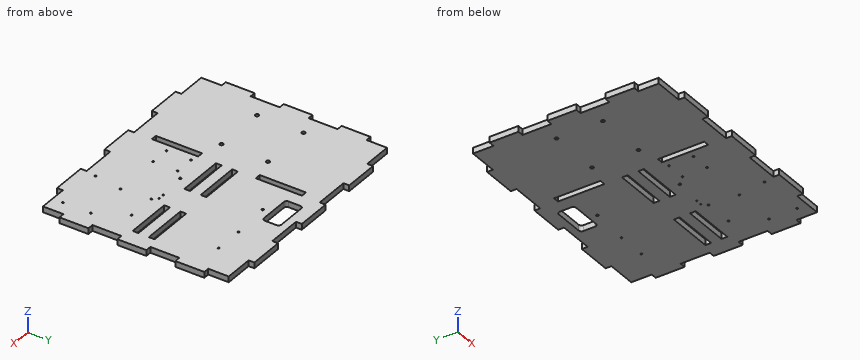
```python
from build123d import *

# Parameters (mm, degrees)
SKETCH_W        = 10
SKETCH_H        = 79.8
SKETCH_W_2      = 79.8
SKETCH_H_2      = 10
PAD_DEPTH       = 10
SKETCH001_R     = 3
POCKET_DEPTH    = 10.001
SKETCH002_R     = 1.5
POCKET001_DEPTH = 10.001
SKETCH003_R     = 1.5
POCKET002_DEPTH = 10.001
SKETCH004_R     = 2
POCKET003_DEPTH = 10.001
POCKET004_DEPTH = 10.001
SKETCH006_R     = 1.2
POCKET005_DEPTH = 10.001
SKETCH007_R     = 1.5
POCKET006_DEPTH = 10.001


with BuildPart() as part:
    # Sketch → Pad (new body)
    with BuildSketch(Plane.XY):
        Polygon((0, 0), (0, 35.3), (-10, 35.3), (-10, 85.1), (0, 85.1), (0, 135.1), (-10, 135.1), (-10, 184.9), (0, 184.9), (0, 234.9), (-10, 234.9), (-10, 284.7), (0, 284.7), (0, 320), (50.2, 320), (50.2, 330), (110.2, 330), (110.2, 320), (170.2, 320), (170.2, 330), (230.2, 330), (230.2, 320), (290.2, 320), (290.2, 330), (350.2, 330), (350.2, 320), (400.4, 320), (400.4, 284.7), (410.4, 284.7), (410.4, 234.9), (400.4, 234.9), (400.4, 184.9), (410.4, 184.9), (410.4, 135.1), (400.4, 135.1), (400.4, 85.1), (410.4, 85.1), (410.4, 35.3), (400.4, 35.3), (400.4, 0), (350.2, 0), (350.2, -10), (290.2, -10), (290.2, 0), (230.2, 0), (230.2, -10), (170.2, -10), (170.2, 0), (110.2, 0), (110.2, -10), (50.2, -10), (50.2, 0), align=None)
        with Locations((165, 249.5)):
            Rectangle(SKETCH_W, SKETCH_H, mode=Mode.SUBTRACT)
        with Locations((165, 70.5)):
            Rectangle(SKETCH_W, SKETCH_H, mode=Mode.SUBTRACT)
        with Locations((209.9, 174)):
            Rectangle(SKETCH_W_2, SKETCH_H_2, mode=Mode.SUBTRACT)
        with Locations((340.9, 174)):
            Rectangle(SKETCH_W_2, SKETCH_H_2, mode=Mode.SUBTRACT)
        with Locations((209.9, 146)):
            Rectangle(SKETCH_W_2, SKETCH_H_2, mode=Mode.SUBTRACT)
        with Locations((340.7, 146)):
            Rectangle(SKETCH_W_2, SKETCH_H_2, mode=Mode.SUBTRACT)
    extrude(amount=PAD_DEPTH)

    # Sketch001 (on DatumPlane) → Pocket (cut, through all)
    with BuildSketch(Plane.XY.offset(10)):
        with Locations((35, 120)):
            Circle(SKETCH001_R)
        with Locations((125, 120)):
            Circle(SKETCH001_R)
        with Locations((125, 200)):
            Circle(SKETCH001_R)
        with Locations((35, 200)):
            Circle(SKETCH001_R)
    extrude(amount=-POCKET_DEPTH, mode=Mode.SUBTRACT)

    # Sketch002 (on DatumPlane) → Pocket001 (cut, through all)
    with BuildSketch(Plane.XY.offset(10)):
        with Locations((298, 267)):
            Circle(SKETCH002_R)
        with Locations((348, 267)):
            Circle(SKETCH002_R)
        with Locations((298, 117)):
            Circle(SKETCH002_R)
        with Locations((348, 117)):
            Circle(SKETCH002_R)
    extrude(amount=-POCKET001_DEPTH, mode=Mode.SUBTRACT)

    # Sketch003 (on DatumPlane) → Pocket002 (cut, through all)
    with BuildSketch(Plane.XY.offset(10)):
        with Locations((376.383, 66.166)):
            Circle(SKETCH003_R)
        with Locations((376.383, 17.83)):
            Circle(SKETCH003_R)
        with Locations((293.757, 17.83)):
            Circle(SKETCH003_R)
        with Locations((301.25, 66.166)):
            Circle(SKETCH003_R)
    extrude(amount=-POCKET002_DEPTH, mode=Mode.SUBTRACT)

    # Sketch004 (on DatumPlane) → Pocket003 (cut, through all)
    with BuildSketch(Plane.XY.offset(10)):
        with Locations((231, 263)):
            Circle(SKETCH004_R)
        with Locations((231, 121)):
            Circle(SKETCH004_R)
    extrude(amount=-POCKET003_DEPTH, mode=Mode.SUBTRACT)

    # Sketch005 (on DatumPlane) → Pocket004 (cut, through all)
    with BuildSketch(Plane.XY.offset(10)):
        with BuildLine():
            Line((198, 307), (248, 307))
            ThreePointArc((253, 302), (251.535534, 305.535534), (248, 307))
            Line((253, 302), (253, 282))
            ThreePointArc((248, 277), (251.535534, 278.464466), (253, 282))
            Line((248, 277), (198, 277))
            ThreePointArc((193, 282), (194.464466, 278.464466), (198, 277))
            Line((193, 282), (193, 302))
            ThreePointArc((198, 307), (194.464466, 305.535534), (193, 302))
        make_face()
    extrude(amount=-POCKET004_DEPTH, mode=Mode.SUBTRACT)

    # Sketch006 (on DatumPlane) → Pocket005 (cut, through all)
    with BuildSketch(Plane.XY.offset(10)):
        with Locations((279.75, 125)):
            Circle(SKETCH006_R)
        with Locations((290.25, 125)):
            Circle(SKETCH006_R)
    extrude(amount=-POCKET005_DEPTH, mode=Mode.SUBTRACT)

    # Sketch007 (on DatumPlane) → Pocket006 (cut, through all)
    with BuildSketch(Plane.XY.offset(10)):
        with Locations((183, 106.9)):
            Circle(SKETCH007_R)
        with Locations((217, 106.9)):
            Circle(SKETCH007_R)
        with Locations((217, 64.9)):
            Circle(SKETCH007_R)
        with Locations((183, 64.9)):
            Circle(SKETCH007_R)
    extrude(amount=-POCKET006_DEPTH, mode=Mode.SUBTRACT)


solid = part.part
```
Check sheet for the modelled part. Datum: model origin and axes. Units: mm. Round coordinates to 2 decimals unless told otherwise and drop trailing zeros. Loops run counter-clockwise (first coordinate to the right, second up) from the corner with the lowest first, then second, coordinate; pieces in that order, holes last. Notation, with made-up numbers: (33, 22) - (49, 22) arc R16 cw to (49, 51) - close; hole circle Ø11 at (50.5, -36.75). An arc over 180 degrees is marked (long way). Answer as a JSON object with one key per item and string values. Group by question number.
Q1. Scan lines: line 1 along Y through (x, z) = (183, 2.25); line 2 along Y through (x, z) = (352, 4); line 3 along Y through (x, z) = (298, 7.75). Record each from-to range of solid material in increasing order. Write a range as [from, to].
Q2. Gauge pin test, flat ends, axial feed: P1, Ø5, axis at x = -7.5, z = 7, coming from the -Y side; P2, Ø3, axis at x = 405, z = 6, coming from the +Y side; P3, Ø3, axis at x = 166, z = 6.5, coming from the +Y side. Record the tip position at first contact, or that the pin passes through.
Q3. Sectioned sample at A-A, the plane y = 98. Enter the section's corners in (x, z).
Q4. Sectioned sample at B-B, the plane x = 327. Enter the section's corners in (y, z).
Q5. Sectioned sample at C-C, the plane z = 2.5. Count the separate pieces of the cut face and the enclosed holes in it, plus the area to 3 significant figures.
Solution:
{
 "1": {"line 1": "y = [-10, 63.4], [66.4, 105.4], [108.4, 141], [151, 169], [179, 330]", "line 2": "y = [0, 141], [151, 169], [179, 320]", "line 3": "y = [-10, 115.5], [118.5, 265.5], [268.5, 330]"},
 "2": {"P1": "stops at y = 35.3", "P2": "stops at y = 284.7", "P3": "stops at y = 320"},
 "3": {"outline": "(0, 0) - (160, 0) - (160, 10) - (0, 10) - close; (170, 0) - (400.4, 0) - (400.4, 10) - (170, 10) - close"},
 "4": {"outline": "(-10, 0) - (141, 0) - (141, 10) - (-10, 10) - close; (151, 0) - (169, 0) - (169, 10) - (151, 10) - close; (179, 0) - (330, 0) - (330, 10) - (179, 10) - close"},
 "5": {"separate pieces": "1", "enclosed holes": "27", "area": "128,000 mm²"}
}
